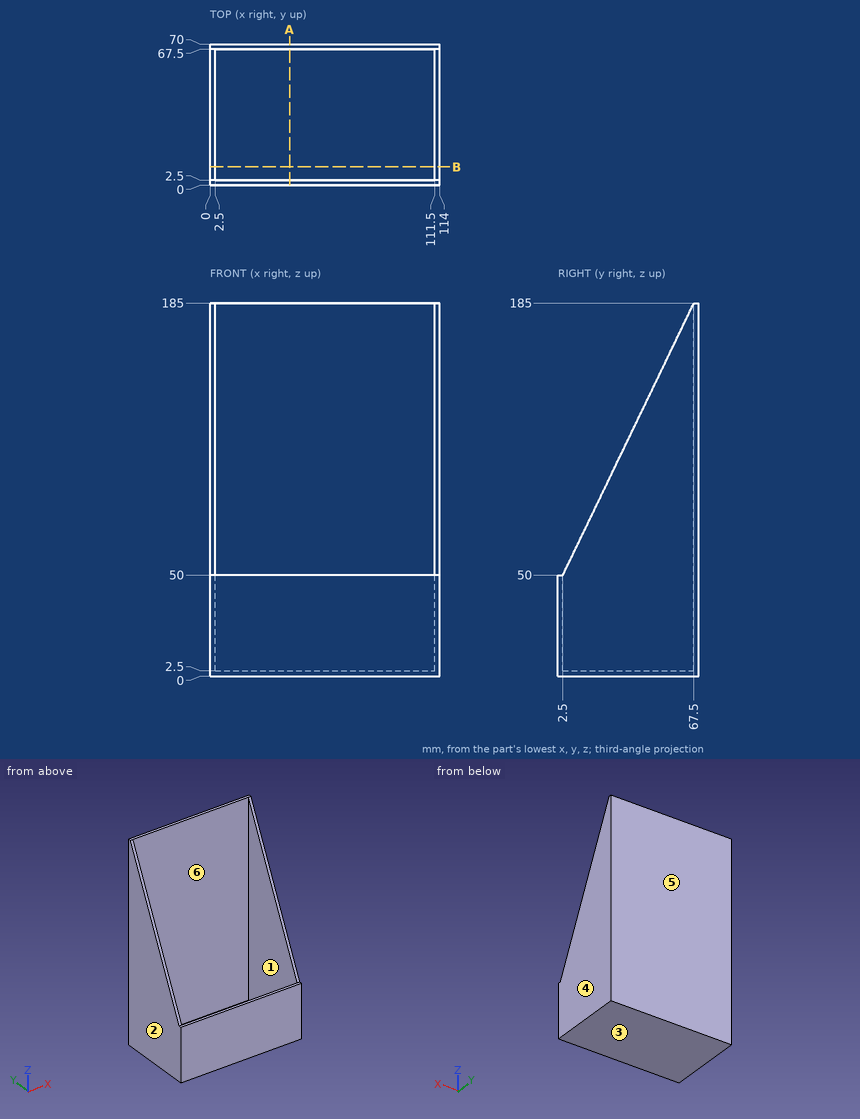
Here's the drawing with two shaded views (mm, measured from the low corner). I have some questions. A direction names the side the tool comes from. Coordinates: 2 decimals unless noted, no trailing zeros. Order: outer loops, then holes, each group sorted by start corner. A loop starts at its lowest first (then second) coordinate and runs counter-clockwise, first axis right, second up.
Q1. Will these pins go through, and if not, where does the flat tip stop? pin 1 (2 mm diameter, centred on y = 21, z = 93.5, fed in from -X); pin 2 (0.8 mm diameter, centred on x = 69.5, y = 1, fed in from +Z); pin 3 (12 mm diameter, centred on x = 31, z = 103, fed in from -Y); pin 4 (1.5 mm diameter, centred on x = 70.5, y = 38.5, fed in from +Z).
Q2. Please list where these lines run through material, in increasing order: L1, parallel to X at y = 61.5, z = 80.5; L2, parallel to Z at x = 95, y = 30.5; L3, parallel to Y at x = 104.5, z = 20.
Q3. Suppose I cut it at A-A on x = 39.5. Please give me the cut outline in (y, z).
Q4. Thinking about a two-plate mould opening in X: for the marked faces 1, 2, 3 and 4, which applies, released by +X, released by -X, zero draft, split by the parting line, or undercut?
Q5. Suppose I cut it at B-B on y = 9. Please give me the cut outline in (x, z), and give its area (3 significant figures).
Q6. Which directions (+Z, -Z, +X, -X, +Y, -Y) give clear straight access to the entire face, cutting with the end or side of a thin tool? Please do the marked faces 5 and 6.
Answer:
1. pin 1: passes through
1. pin 2: stops at z = 50
1. pin 3: stops at y = 67.5
1. pin 4: stops at z = 2.5
2. L1: x = 0 to 2.5, 111.5 to 114
2. L2: z = 0 to 2.5
2. L3: y = 0 to 2.5, 67.5 to 70
3. outline: (0, 0) - (70, 0) - (70, 185) - (67.5, 185) - (67.5, 2.5) - (2.5, 2.5) - (2.5, 50) - (0, 50) - close
4. face 1: undercut
4. face 2: released by -X
4. face 3: zero draft
4. face 4: released by +X
5. outline: (0, 0) - (114, 0) - (114, 63.5) - (111.5, 63.5) - (111.5, 2.5) - (2.5, 2.5) - (2.5, 63.5) - (0, 63.5) - close
5. area: 590 mm2
6. face 5: +Z, -Z, +X, -X, +Y
6. face 6: +Z
